The figure shows three views and two pictorial views of one solid part (mm, origin at its lowest corner). Answer the questions. Give positions to 0.01 mm unless a question says otherwise; leave off trailing zeros. Order: outer loops, then holes, each group sorted by start corner. A loop starts at its lowest first (then second) coordinate and runs counter-clockwise, first axis right, second up. Notation, with made-up numbers: (-4, 10) - (51, 10) arc R31 ccw to (51, 47) - close; hole circle Ø4 at (-7.5, 20). An arc over 180 degrees is marked (long way). Use a Markdown table: item, result. Add a question column.
1. A cutting plane is placed at C-C on y = 23. Determine the outline of the cut face in (x, z) (1 decimal).
2. Consider L1, parallel to Y at x = 1.4, z = 63.5; L2, parallel to Y at x = 0.45, z = 38; L3, parallel to Y at x = 1.6, z = 12 (1 decimal). Determine where each line is inside the solid, lowest interval first.
3. A cutting plane is placed at B-B on z = 67. Determine the outline of the cut face in (x, y) (1 decimal), and give its area (3 significant figures).
4. A flat-ended cylindrical pin translates along its axis: P1, Ø1, axis at x = 1.5, y = 66, coming from the +Z side. Find the tip coordinate at first contact, or state that the pin passes through.
5. A cutting plane is placed at A-A on x = 2.6. Determine the outline of the cut face in (y, z) (1 decimal), and give its area (3 significant figures).
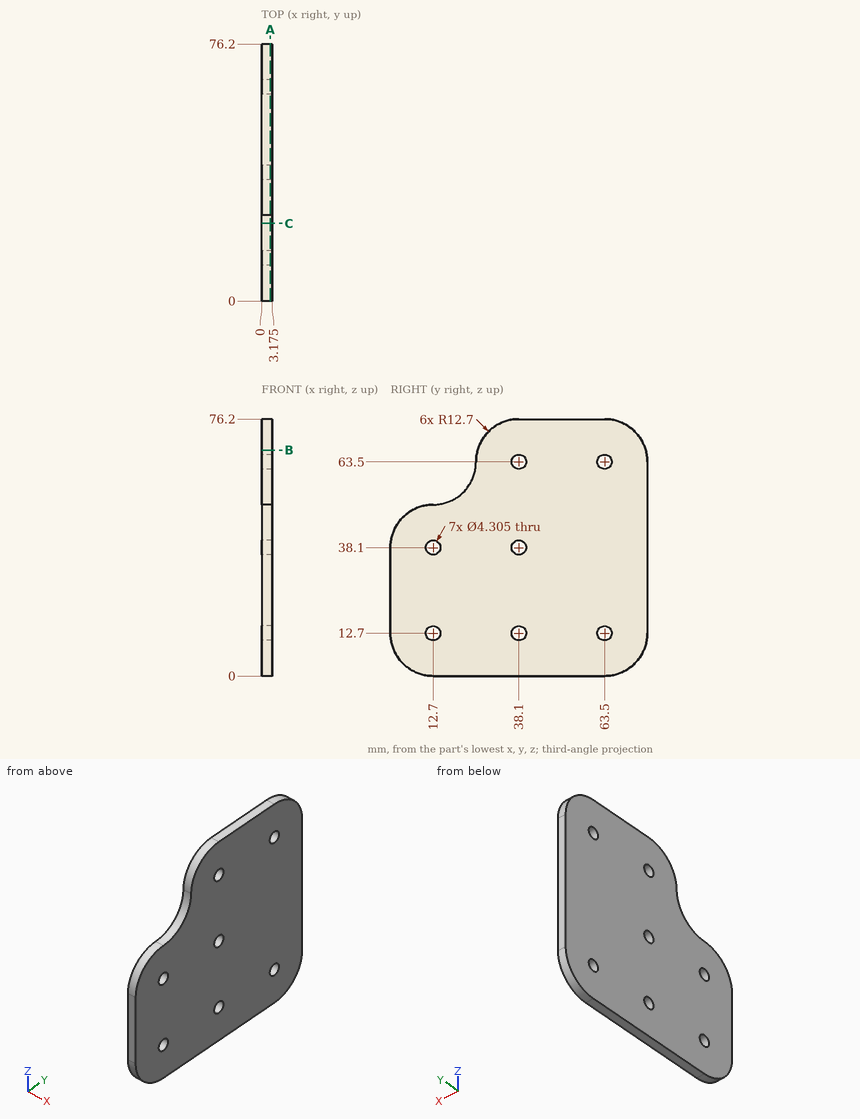
Output values:
| question | item | result |
|---|---|---|
| 1 | outline | (0, 0) - (3.2, 0) - (3.2, 56.1) - (0, 56.1) - close |
| 2 | L1 | 25.4 to 35.95, 40.25 to 61.35, 65.65 to 76.2 |
| 2 | L2 | 0 to 10.55, 14.85 to 35.95, 40.25 to 76.2 |
| 2 | L3 | 0 to 10.7, 14.7 to 36.1, 40.1 to 61.5, 65.5 to 76.2 |
| 3 | outline | (0, 25.9) - (3.2, 25.9) - (3.2, 75.7) - (0, 75.7) - close |
| 3 | area | 158 mm² |
| 4 | P1 | z = 76.04 |
| 5 | outline | (0, 12.7) arc R12.7 ccw to (12.7, 0) - (63.5, 0) arc R12.7 ccw to (76.2, 12.7) - (76.2, 63.5) arc R12.7 ccw to (63.5, 76.2) - (38.1, 76.2) arc R12.7 ccw to (25.4, 63.5) arc R12.7 cw to (12.7, 50.8) arc R12.7 ccw to (0, 38.1) - close; hole circle Ø4.3 at (12.7, 12.7); hole circle Ø4.3 at (12.7, 38.1); hole circle Ø4.3 at (38.1, 12.7); hole circle Ø4.3 at (38.1, 38.1); hole circle Ø4.3 at (38.1, 63.5); hole circle Ø4.3 at (63.5, 12.7); hole circle Ø4.3 at (63.5, 63.5) |
| 5 | area | 4,920 mm² |
